```python
from build123d import *

# Parameters (mm, degrees)
SKETCH1_R           = 8
BOSS_EXTRUDE1_DEPTH = 30
SKETCH2_R           = 8
BOSS_EXTRUDE2_DEPTH = 1
BOSS_EXTRUDE2_TAPER = 45
SKETCH3_R           = 6
BOSS_EXTRUDE3_DEPTH = 3
SKETCH4_W           = 6
SKETCH4_H           = 6
BOSS_EXTRUDE4_DEPTH = 3
BOSS_EXTRUDE5_DEPTH = 20
SKETCH9_R           = 2.05
CUT_EXTRUDE1_DEPTH  = 6


with BuildPart() as part:
    # Sketch1 → Boss-Extrude1 (new body)
    with BuildSketch(Plane(origin=(0, 0, 0), x_dir=(1, 0, 0), z_dir=(0, 1, 0))):
        with Locations(Location((0, 0, 0), (0, 0, 270))):
            Circle(SKETCH1_R)
    extrude(amount=BOSS_EXTRUDE1_DEPTH)

    # Sketch2 → Boss-Extrude2 (add)
    with BuildSketch(Plane(origin=(0, 30, 0), x_dir=(1, 0, 0), z_dir=(0, 1, 0))):
        with Locations(Location((0, 0, 0), (0, 0, 270))):
            Circle(SKETCH2_R)
    extrude(amount=BOSS_EXTRUDE2_DEPTH, taper=BOSS_EXTRUDE2_TAPER)

    # Sketch3 → Boss-Extrude3 (add)
    with BuildSketch(Plane(origin=(0, 31, 0), x_dir=(1, 0, 0), z_dir=(0, 1, 0))):
        with Locations(Location((0, 0, 0), (0, 0, 270))):
            Circle(SKETCH3_R)
    extrude(amount=BOSS_EXTRUDE3_DEPTH)

    # Sketch4 → Boss-Extrude4 (add)
    with BuildSketch(Plane(origin=(0, 34, 0), x_dir=(1, 0, 0), z_dir=(0, 1, 0))):
        Rectangle(SKETCH4_W, SKETCH4_H)
    extrude(amount=BOSS_EXTRUDE4_DEPTH)

    # Sketch6 for Loft1 → Loft1 section 0
    with BuildSketch(Plane(origin=(0, 43, 0), x_dir=(1, 0, 0), z_dir=(0, 1, 0))):
        with BuildLine():
            # circular arc as an exact rational Bezier (weights 1, cos(half-angle), 1)
            Bezier((4.949747468, -4.949747468), (9.899494937, 0), (4.949747468, 4.949747468), weights=[1, 0.707106781, 1])
            Bezier((4.949747468, 4.949747468), (0, 9.899494937), (-4.949747468, 4.949747468), weights=[1, 0.707106781, 1])
            Bezier((-4.949747468, 4.949747468), (-9.899494937, 0), (-4.949747468, -4.949747468), weights=[1, 0.707106781, 1])
            Bezier((-4.949747468, -4.949747468), (0, -9.899494937), (4.949747468, -4.949747468), weights=[1, 0.707106781, 1])
        make_face()
    # Sketch5 → Loft1 section 1
    with BuildSketch(Plane(origin=(0, 37, 0), x_dir=(1, 0, 0), z_dir=(0, 1, 0))):
        with BuildLine():
            Line((3, -3), (3, 3))
            Line((3, 3), (-3, 3))
            Line((-3, 3), (-3, -3))
            Line((-3, -3), (3, -3))
        make_face()
    loft()

    # Sketch7 → Boss-Extrude5 (add)
    with BuildSketch(Plane(origin=(0, 43, 0), x_dir=(1, 0, 0), z_dir=(0, 1, 0))):
        with BuildLine():
            ThreePointArc((4.949747468, -4.949747468), (7, 0), (4.949747468, 4.949747468))
            ThreePointArc((4.949747468, 4.949747468), (0, 7), (-4.949747468, 4.949747468))
            ThreePointArc((-4.949747468, 4.949747468), (-7, 0), (-4.949747468, -4.949747468))
            ThreePointArc((-4.949747468, -4.949747468), (0, -7), (4.949747468, -4.949747468))
        make_face()
    extrude(amount=BOSS_EXTRUDE5_DEPTH)

    # Fillet1: read off the stored shape, not the designer's step
    # Fillet1 outline → Fillet1 (revolve, cut)
    with BuildSketch(Plane.XY):
        with BuildLine():
            ThreePointArc((1, 63), (5.242640687, 61.242640687), (7, 57))
            Line((7, 57), (7, 63))
            Line((7, 63), (1, 63))
        make_face()
    revolve(axis=Axis((0, 0, 0), (0, 1, 0)), mode=Mode.SUBTRACT)

    # Sketch9 → Cut-Extrude1 (cut)
    with BuildSketch(Plane.XZ):
        with Locations(Location((0, 0, 0), (0, 0, 270))):
            Circle(SKETCH9_R)
    extrude(amount=-CUT_EXTRUDE1_DEPTH, mode=Mode.SUBTRACT)


solid = part.part
```
Can you work these out from the model? Positions are in its coordinate system, mm. A direction names the side the tool comes from. Give positions to 0.01 mm unless a question says otherwise; leave off trailing zeros. Loops run counter-clockwise (first coordinate to the right, second up) from the corner with the lowest first, then second, coordinate; pieces in that order, holes last. Notation, with made-up numbers: M 43.25,83.25 L 58.25,83.25 A21 ccw 58.25,93.25 Z; hole C 18,82.5 d10. An arc over 180 degrees is marked long. One line per item, written item: value.
(1) Which directions (+Z, -Z, +X, -X, +Y, -Y) give clear straight access to the entire face, cutting with the end or side of a thin tool? Please do faces 1 (the face through (-4, 34, 0)), 2 (the face through (0, 35, 3)), 3 (the face through (3, 35, 0)).
Returned:
face 1: none
face 2: +Z, +X, -X
face 3: +Z, -Z, +X
(2) We'd pull the mould along X, two halves only. Please class faces 4 (the face through (0, 35, -3)), 5 (the face through (2.033, 2.958, 0.267)), 6 (the face through (0, 6, 0)), 7 (the face through (-7.81, 14.79, -1.73)): released by +X, released by -X, zero draft, split by the parting line, or undercut.
Returned:
face 4: zero draft
face 5: undercut
face 6: undercut
face 7: split by the parting line
(3) Suppose I cut it at A-A on y = 9. List the corners of the cut face in (x, z) for me.
Returned:
outline: C 0,0 d16
(4) I need wall thicknesses on line 1 (X direction, y = 1.8, z = 0); line 2 (Y direction, x = -5.25, z = -2.5); line 3 (Y direction, x = 6, z = -0.75). Which ranges of each line are inside material? Lowest first, please.
Returned:
line 1: -8 to -2.05, 2.05 to 8
line 2: 0 to 34, 41.03 to 60.58
line 3: 0 to 31, 41.56 to 60.25
(5) Will these pins go through, and if not, where does the flat tip stop? pin 1 (2 mm diameter, centred on x = -6, y = 18, fed in from +Z) (3 decimals); pin 2 (3.5 mm diameter, centred on y = 36, z = 1, fed in from +X); pin 3 (3.5 mm diameter, centred on x = -1, y = 35.5, fed in from +Z).
Returned:
pin 1: z = 6.245
pin 2: x = 3.48
pin 3: z = 6
